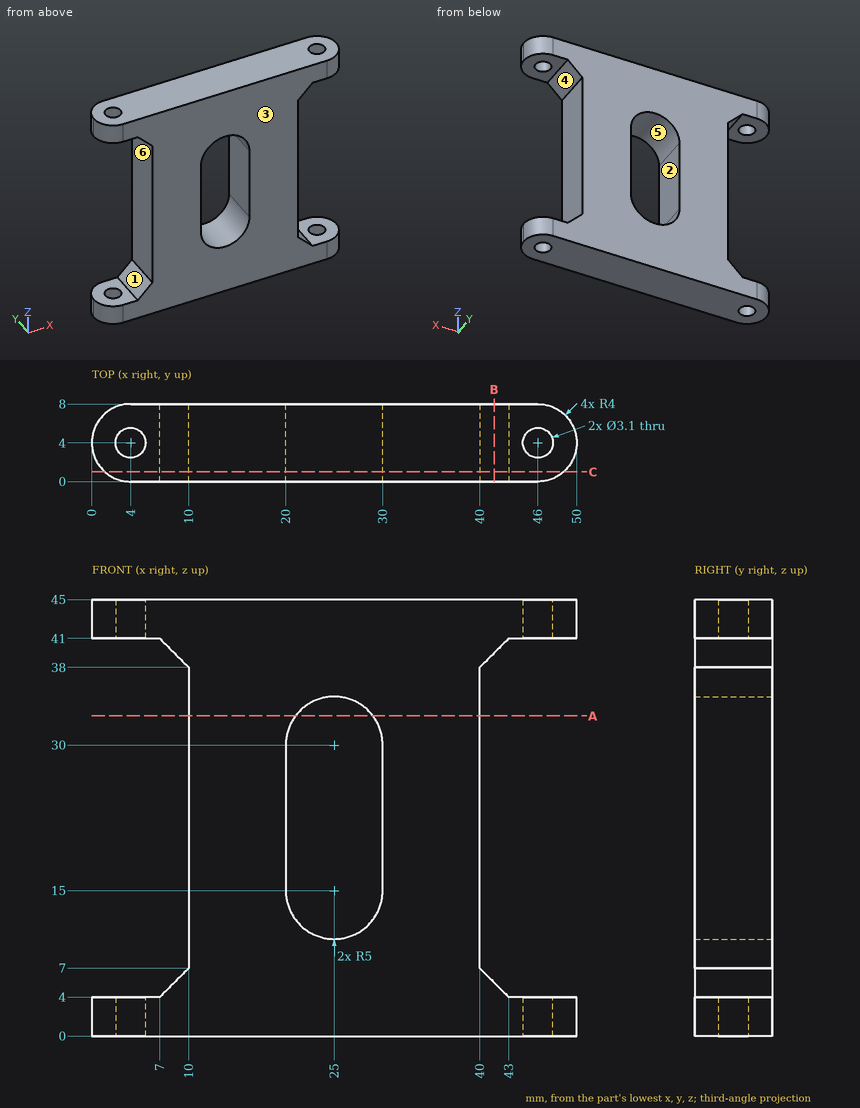
Input: dimensioned drawing with shaded views. Units: mm. Origin: part minimum x, y, z. A direction names the side the tool comes from. Give positions to 0.01 mm unless a question says otherwise; leave off trailing zeros. Write each loop counter-clockwise with the first axis right and the second up, starting at its lowest first coordinate (ties: lowest second). Pieces come first, ordered by that corner, then holes. Notation, with made-up numbers: (75, -27) -> (86, -27) arc R19 cw to (86, -6) -> close; hole circle Ø7 at (10.5, 66). An arc over 180 degrees is marked (long way). Return JSON: item names as keys, results as strings. Group by question number.
1. Section A-A, the plane z = 33. Output: boundary loops of the cut face in (x, y), then the cut area to 3 significant figures.
2. Pin query (flat end, axial travel): pin 1 Ø2 at (y, z) = (6.5, 39.5) entering from +X; pin 2 Ø2 at (y, z) = (3, 6) entering from +X; pin 3 Ø4 at (y, z) = (3, 21.5) entering from -X. Return the tip coordinate at first contact, or that it passes through.
3. Material intervals for line 1 (X direction, y = 4, z = 42.4); line 2 (Y direction, x = 4, z = 1.65); line 3 (Z direction, x = 25, y = 2.25), sorted ascending. Write a range as from..to.
4. Access query for the marked faces 4, 5 and 6. Directions: +Z, -Z, +X, -X, +Y, -Y. A direction counts if a zero-diameter tool reaches every point of the face in a straight line with its end or side. Return the directions, or none.
5. Section C-C, the plane y = 1. Output: boundary loops of the cut face in (x, z).
6. Section B-B, the plane x = 41.5. Output: boundary loops of the cut face in (y, z).
7. Mould query, pull axis X, two halves, no side actions, for the marked faces 1, 2 and 3. Classes: +X half, -X half, draft (parallel to the pull), parting line (faces both ways), or undercut.
Determined:
{
 "1": {"outline": "(10, 0) -> (21, 0) -> (21, 8) -> (10, 8) -> close; (29, 0) -> (40, 0) -> (40, 8) -> (29, 8) -> close", "area": "176 mm2"},
 "2": {"pin 1": "stops at x = 42.5", "pin 2": "stops at x = 42", "pin 3": "stops at x = 10"},
 "3": {"line 1": "x = 0..2.45, 5.55..44.45, 47.55..50", "line 2": "y = 0..2.45, 5.55..8", "line 3": "z = 0..10, 35..45"},
 "4": {"face 4": "+X, +Y, -Y", "face 5": "+Y, -Y", "face 6": "-X, +Y, -Y"},
 "5": {"outline": "(1.35, 0) -> (48.65, 0) -> (48.65, 4) -> (43, 4) -> (40, 7) -> (40, 38) -> (43, 41) -> (48.65, 41) -> (48.65, 45) -> (1.35, 45) -> (1.35, 41) -> (7, 41) -> (10, 38) -> (10, 7) -> (7, 4) -> (1.35, 4) -> close; hole (20, 15) arc R5 ccw to (30, 15) -> (30, 30) arc R5 ccw to (20, 30) -> close"},
 "6": {"outline": "(0, 0) -> (8, 0) -> (8, 5.5) -> (0, 5.5) -> close; (0, 39.5) -> (8, 39.5) -> (8, 45) -> (0, 45) -> close"},
 "7": {"face 1": "-X half", "face 2": "undercut", "face 3": "draft"}
}
